For this review, use the dimensioned drawing (mm, ordinates from the lowest corner) and the shaded views. Give positions to 0.01 mm unless a question says otherwise; leave off trailing zeros. Order: outer loops, then holes, each group sorted by start corner. A loop starts at its lowest first (then second) coordinate and runs counter-clockwise, first axis right, second up. Notation, with made-up numbers: (29.5, 77) - (34.5, 77) arc R23 ccw to (34.5, 111) - close; hole circle Ø11 at (73.5, 43). An arc over 180 degrees is marked (long way). One line per item, written item: value.
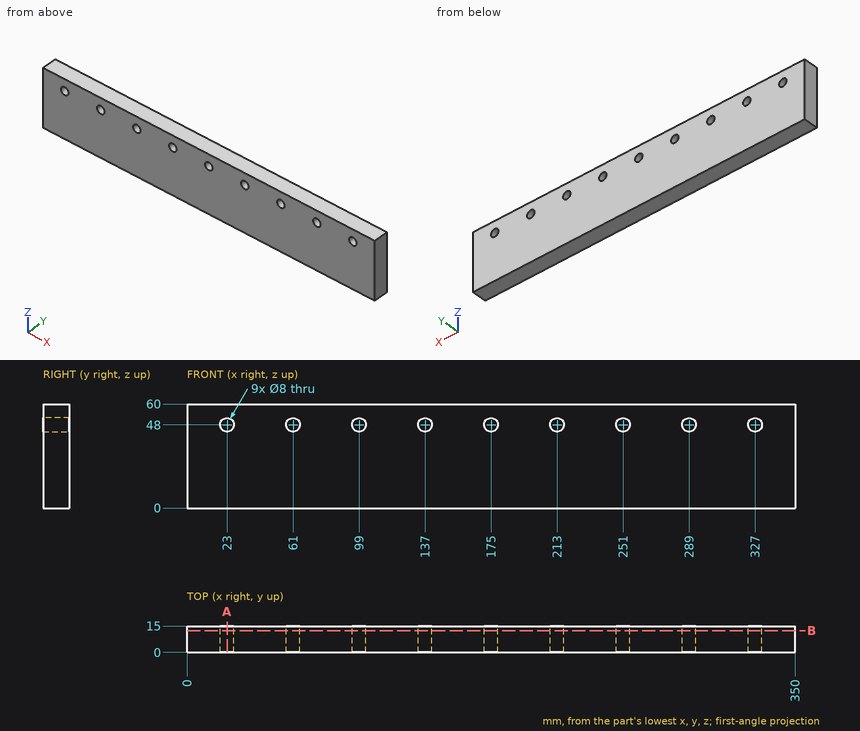
(1) For P1, Ø4, axis at y = 2.5, z = 14.5, coming from the -X side; P2, Ø7, axis at x = 23, z = 48, coming from the -Y side, all flat-tipped, find the tip position at first contact; note any pin that passes through.
Answers below:
P1: stops at x = 0
P2: passes through
(2) Wall thickness on line 1 (Z direction, x = 288.5, y = 8); line 2 (Z direction, x = 138.5, y = 2.5): over which ranges is each line inside the solid? List them lowest first. Write a range as from..to.
Answers below:
line 1: z = 0..44.03, 51.97..60
line 2: z = 0..44.29, 51.71..60
(3) Take a section at A-A (x = 23). Write out the cut boundary in (y, z).
Answers below:
outline: (0, 0) - (15, 0) - (15, 44) - (0, 44) - close; (0, 52) - (15, 52) - (15, 60) - (0, 60) - close
(4) Take a section at B-B (y = 12.5). Give the number of separate pieces and of enclosed holes in the cut face, then the cut area to 3 significant figures.
Answers below:
separate pieces: 1
enclosed holes: 9
area: 20,500 mm^2
